Input: part model. Units: mm. Frame: model coordinates. A direction names the side the tool comes from. Round coordinates to 2 decimals unless told otherwise and drop trailing zeros. Order: outer loops, then holes, each group sorted by start corner. A loop starts at its lowest first (then second) coordinate and runs counter-clockwise, first axis right, second up. Notation, with made-up numbers: (-34, 25) -> (3, 25) arc R21 ccw to (3, 57) -> close; hole circle Ø1 at (-14, 8). An arc over 180 degrees is marked (long way). Use a Markdown table: item, result.
from build123d import *

# Parameters (mm, degrees)
SKETCH1_W           = 125
SKETCH1_H           = 60
SKETCH1_R           = 2.8
SKETCH1_R_2         = 3.25
SKETCH1_R_3         = 2.75
BOSS_EXTRUDE1_DEPTH = 30
CUT_EXTRUDE1_DEPTH  = 15
SKETCH3_R           = 3.25
CUT_EXTRUDE2_DEPTH  = 19
BOSS_EXTRUDE2_DEPTH = 5
BOSS_EXTRUDE3_REACH = 143.863
SKETCH5_W           = 6
SKETCH5_H           = 60
SKETCH5_H_2         = 17.5
SKETCH5_H_3         = 7.275
SKETCH5_W_2         = 3
SKETCH5_W_3         = 10
SKETCH5_H_4         = 15
CUT_EXTRUDE3_DEPTH  = 148.564392724
SKETCH7_W           = 23
SKETCH7_H           = 18
BOSS_EXTRUDE4_DEPTH = 12.5
SKETCH8_R           = 3.25
CUT_EXTRUDE4_DEPTH  = 129.082004981
SKETCH9_R           = 2.7
SKETCH9_W           = 24
SKETCH9_H           = 15.5
SKETCH9_W_2         = 46
BOSS_EXTRUDE5_DEPTH = 5
SKETCH10_R          = 2.7
BOSS_EXTRUDE6_DEPTH = 5
SKETCH11_R          = 2.6
CUT_EXTRUDE5_DEPTH  = 158.877325794
SKETCH12_R          = 3.5
SKETCH12_R_2        = 2.8
BOSS_EXTRUDE7_DEPTH = 0.75
FILLET1_R           = 0.75


with BuildPart() as part:
    # Sketch1 → Boss-Extrude1 (new body)
    with BuildSketch(Plane.XY):
        with Locations((-62.5, 30)):
            Rectangle(SKETCH1_W, SKETCH1_H)
        with Locations((-42.5, 42.725)):
            Circle(SKETCH1_R, mode=Mode.SUBTRACT)
        with Locations((-22, 30)):
            Circle(SKETCH1_R, mode=Mode.SUBTRACT)
        with Locations((-15, 45)):
            Circle(SKETCH1_R_2, mode=Mode.SUBTRACT)
        with Locations((-15, 15)):
            Circle(SKETCH1_R_2, mode=Mode.SUBTRACT)
        with Locations((-115, 15)):
            Circle(SKETCH1_R_3, mode=Mode.SUBTRACT)
        with Locations((-115, 45)):
            Circle(SKETCH1_R_3, mode=Mode.SUBTRACT)
    extrude(amount=BOSS_EXTRUDE1_DEPTH)

    # Sketch2 → Cut-Extrude1 (cut)
    with BuildSketch(Plane.XY.offset(30)):
        with BuildLine():
            Line((0, 0), (-22.5, 0))
            Line((-22.5, 0), (-22.5, 17.5))
            ThreePointArc((-22.5, 17.5), (-21.035533906, 21.035533906), (-17.5, 22.5))
            Line((-17.5, 22.5), (0, 22.5))
            Line((0, 22.5), (0, 0))
        make_face()
        with BuildLine():
            Line((0, 60), (-22.5, 60))
            Line((-22.5, 60), (-22.5, 42.5))
            ThreePointArc((-22.5, 42.5), (-21.035533906, 38.964466094), (-17.5, 37.5))
            Line((-17.5, 37.5), (0, 37.5))
            Line((0, 37.5), (0, 60))
        make_face()
        with BuildLine():
            Line((-107.5, 60), (-107.5, 42.5))
            ThreePointArc((-107.5, 42.5), (-108.964466094, 38.964466094), (-112.5, 37.5))
            Line((-112.5, 37.5), (-125, 37.5))
            Line((-125, 37.5), (-125, 60))
            Line((-125, 60), (-107.5, 60))
        make_face()
        with BuildLine():
            Line((-125, 0), (-107.5, 0))
            Line((-107.5, 0), (-107.5, 17.5))
            ThreePointArc((-107.5, 17.5), (-108.964466094, 21.035533906), (-112.5, 22.5))
            Line((-112.5, 22.5), (-125, 22.5))
            Line((-125, 22.5), (-125, 0))
        make_face()
    extrude(amount=-CUT_EXTRUDE1_DEPTH, mode=Mode.SUBTRACT)

    # Sketch3 → Cut-Extrude2 (cut)
    with BuildSketch(Plane(origin=(0, 0, 0), x_dir=(-1, 0, 0), z_dir=(0, 0, -1))):
        with Locations((22, 30)):
            Circle(SKETCH3_R)
        with Locations((42.5, 42.725)):
            Circle(SKETCH3_R)
    extrude(amount=-CUT_EXTRUDE2_DEPTH, mode=Mode.SUBTRACT)


with BuildPart() as body_2:
    # Sketch4 → Boss-Extrude2 (new body)
    with BuildSketch(Plane.XY.offset(45.5)):
        with BuildLine():
            Line((-107.5, 60), (-107.5, 0))
            Line((-107.5, 0), (-22.5, 0))
            Line((-22.5, 0), (-22.5, 17.5))
            ThreePointArc((-22.5, 17.5), (-21.035533906, 21.035533906), (-17.5, 22.5))
            Line((-17.5, 22.5), (0, 22.5))
            Line((0, 22.5), (0, 37.5))
            Line((0, 37.5), (-17.5, 37.5))
            ThreePointArc((-17.5, 37.5), (-21.035533906, 38.964466094), (-22.5, 42.5))
            Line((-22.5, 42.5), (-22.5, 60))
            Line((-22.5, 60), (-107.5, 60))
        make_face()
    extrude(amount=BOSS_EXTRUDE2_DEPTH)

    # Sketch5 → Boss-Extrude3 (add, up to next)
    with BuildSketch(Plane.XY.offset(30), mode=Mode.PRIVATE) as boss_extrude3_sk1:
        with Locations((-104.5, 30)):
            Rectangle(SKETCH5_W, SKETCH5_H)
    boss_extrude3_tool1 = extrude(boss_extrude3_sk1.sketch, amount=BOSS_EXTRUDE3_REACH, mode=Mode.PRIVATE) - body_2.part
    # Sketch5 → Boss-Extrude3 (add, up to next)
    with BuildSketch(Plane.XY.offset(30), mode=Mode.PRIVATE) as boss_extrude3_sk2:
        with Locations((-25.5, 8.75)):
            Rectangle(SKETCH5_W, SKETCH5_H_2)
    boss_extrude3_tool2 = extrude(boss_extrude3_sk2.sketch, amount=BOSS_EXTRUDE3_REACH, mode=Mode.PRIVATE) - body_2.part
    # Sketch5 → Boss-Extrude3 (add, up to next)
    with BuildSketch(Plane.XY.offset(30), mode=Mode.PRIVATE) as boss_extrude3_sk3:
        with Locations((-25.5, 51.25)):
            Rectangle(SKETCH5_W, SKETCH5_H_2)
    boss_extrude3_tool3 = extrude(boss_extrude3_sk3.sketch, amount=BOSS_EXTRUDE3_REACH, mode=Mode.PRIVATE) - body_2.part
    # Sketch5 → Boss-Extrude3 (add, up to next)
    with BuildSketch(Plane.XY.offset(30), mode=Mode.PRIVATE) as boss_extrude3_sk4:
        with Locations((-55.5, 56.3625)):
            Rectangle(SKETCH5_W, SKETCH5_H_3)
    boss_extrude3_tool4 = extrude(boss_extrude3_sk4.sketch, amount=BOSS_EXTRUDE3_REACH, mode=Mode.PRIVATE) - body_2.part
    # Sketch5 → Boss-Extrude3 (add, up to next)
    with BuildSketch(Plane.XY.offset(30), mode=Mode.PRIVATE) as boss_extrude3_sk5:
        with Locations((-54, 8.75)):
            Rectangle(SKETCH5_W_2, SKETCH5_H_2)
    boss_extrude3_tool5 = extrude(boss_extrude3_sk5.sketch, amount=BOSS_EXTRUDE3_REACH, mode=Mode.PRIVATE) - body_2.part
    # Sketch5 → Boss-Extrude3 (add, up to next)
    with BuildSketch(Plane.XY.offset(30), mode=Mode.PRIVATE) as boss_extrude3_sk6:
        with Locations((-5, 30)):
            Rectangle(SKETCH5_W_3, SKETCH5_H_4)
    boss_extrude3_tool6 = extrude(boss_extrude3_sk6.sketch, amount=BOSS_EXTRUDE3_REACH, mode=Mode.PRIVATE) - body_2.part

    add(part.part)  # Boss-Extrude3 merges part
    add(boss_extrude3_tool1.solids().sort_by_distance((-104.5, 30, 30))[0])
    add(boss_extrude3_tool2.solids().sort_by_distance((-25.5, 8.75, 30))[0])
    add(boss_extrude3_tool3.solids().sort_by_distance((-25.5, 51.25, 30))[0])
    add(boss_extrude3_tool4.solids().sort_by_distance((-55.5, 56.3625, 30))[0])
    add(boss_extrude3_tool5.solids().sort_by_distance((-54, 8.75, 30))[0])
    add(boss_extrude3_tool6.solids().sort_by_distance((-5, 30, 30))[0])

    # Sketch6 → Cut-Extrude3 (cut, through all)
    with BuildSketch(Plane.XY.offset(50.5)):
        with BuildLine():
            Line((-82.5, 41.5), (-75.5, 41.5))
            ThreePointArc((-75.5, 41.5), (-64, 30), (-75.5, 18.5))
            Line((-75.5, 18.5), (-82.5, 18.5))
            ThreePointArc((-82.5, 18.5), (-94, 30), (-82.5, 41.5))
        make_face()
        with BuildLine():
            Line((-91, 43.75), (-98, 43.75))
            ThreePointArc((-98, 43.75), (-99.75, 45.5), (-98, 47.25))
            Line((-98, 47.25), (-91, 47.25))
            ThreePointArc((-91, 47.25), (-89.25, 45.5), (-91, 43.75))
        make_face()
        with BuildLine():
            Line((-67, 47.25), (-60, 47.25))
            ThreePointArc((-60, 47.25), (-58.25, 45.5), (-60, 43.75))
            Line((-60, 43.75), (-67, 43.75))
            ThreePointArc((-67, 43.75), (-68.75, 45.5), (-67, 47.25))
        make_face()
        with BuildLine():
            Line((-91, 12.75), (-98, 12.75))
            ThreePointArc((-98, 12.75), (-99.75, 14.5), (-98, 16.25))
            Line((-98, 16.25), (-91, 16.25))
            ThreePointArc((-91, 16.25), (-89.25, 14.5), (-91, 12.75))
        make_face()
        with BuildLine():
            Line((-67, 16.25), (-60, 16.25))
            ThreePointArc((-60, 16.25), (-58.25, 14.5), (-60, 12.75))
            Line((-60, 12.75), (-67, 12.75))
            ThreePointArc((-67, 12.75), (-68.75, 14.5), (-67, 16.25))
        make_face()
    extrude(amount=-CUT_EXTRUDE3_DEPTH, mode=Mode.SUBTRACT)

    # Sketch7 → Boss-Extrude4 (add)
    with BuildSketch(Plane.XY.offset(50.5)):
        with Locations((-42.5, 30)):
            Rectangle(SKETCH7_W, SKETCH7_H)
    extrude(amount=BOSS_EXTRUDE4_DEPTH)

    # Sketch8 → Cut-Extrude4 (cut, through all)
    with BuildSketch(Plane(origin=(-31, 0, 0), x_dir=(0, 0, -1), z_dir=(1, 0, 0))):
        with Locations((-56.5, 30)):
            Circle(SKETCH8_R)
    extrude(amount=-CUT_EXTRUDE4_DEPTH, mode=Mode.SUBTRACT)

    # Sketch9 → Boss-Extrude5 (add)
    with BuildSketch(Plane.XZ):
        Polygon((-125, 15), (-107.5, 15), (-107.5, 50.5), (-22.5, 50.5), (-22.5, 15), (0, 15), (0, -30), (-125, -30), align=None)
        with Locations((-110, -15)):
            Circle(SKETCH9_R, mode=Mode.SUBTRACT)
        with Locations((-80, -15)):
            Circle(SKETCH9_R, mode=Mode.SUBTRACT)
        with Locations((-45, -15)):
            Circle(SKETCH9_R, mode=Mode.SUBTRACT)
        with Locations((-15, -15)):
            Circle(SKETCH9_R, mode=Mode.SUBTRACT)
        with Locations((-40.5, 37.75)):
            Rectangle(SKETCH9_W, SKETCH9_H, mode=Mode.SUBTRACT)
        with Locations((-78.5, 37.75)):
            Rectangle(SKETCH9_W_2, SKETCH9_H, mode=Mode.SUBTRACT)
    extrude(amount=BOSS_EXTRUDE5_DEPTH)

    # Sketch10 → Boss-Extrude6 (add)
    with BuildSketch(Plane(origin=(0, 0, 0), x_dir=(0, 0, -1), z_dir=(1, 0, 0))):
        Polygon((-50.5, 37.5), (-50.5, 22.5), (-15, 22.5), (-15, -5), (30, -5), (30, 60), (-15, 60), (-15, 37.5), align=None)
        with Locations((15, 45)):
            Circle(SKETCH10_R, mode=Mode.SUBTRACT)
        with Locations((15, 15)):
            Circle(SKETCH10_R, mode=Mode.SUBTRACT)
    extrude(amount=BOSS_EXTRUDE6_DEPTH)

    # Sketch11 → Cut-Extrude5 (cut, through all)
    with BuildSketch(Plane(origin=(0, 0, 45.5), x_dir=(-1, 0, 0), z_dir=(0, 0, -1))):
        with Locations((42.5, 42.725)):
            Circle(SKETCH11_R)
        with Locations((22, 30)):
            Circle(SKETCH11_R)
    extrude(amount=-CUT_EXTRUDE5_DEPTH, mode=Mode.SUBTRACT)

    # Sketch12 → Boss-Extrude7 (add)
    # profile 1 of 2: a face of its own
    with BuildSketch(Plane.XY.offset(30)):
        with Locations((-22, 30)):
            Circle(SKETCH12_R)
        with Locations(Location((-22, 30, 0), (0, 0, 180))):
            Circle(SKETCH12_R_2, mode=Mode.SUBTRACT)
    # profile 2 of 2: a face of its own
    with BuildSketch(Plane.XY.offset(30)):
        with Locations((-42.5, 42.725)):
            Circle(SKETCH12_R)
        with Locations(Location((-42.5, 42.725, 0), (0, 0, 180))):
            Circle(SKETCH12_R_2, mode=Mode.SUBTRACT)
    extrude(amount=BOSS_EXTRUDE7_DEPTH)

    # Fillet1
    fillet1_edges = [body_2.edges().sort_by_distance(p)[0] for p in [
        (-25.5, 30, 30),
        (-46, 42.725, 30),
    ]]
    fillet(fillet1_edges, radius=FILLET1_R - 0.0001)  # a hair under: the kernel refuses the full size


solid = body_2.part
1) Set-up query: faces 4 (the face through (-22.5, 6, 33)), 5 (the face through (-58.5, 56, 38)), 6 (the face through (2.465, 43.966, -17.494)), 7 (the face through (-94, 43.75, 15)). Return all of +Z, -Z, +X, -X, +Y, -Y with unobstructed straight access to the full face (end or side cutting, diameter ignored); none if empty.
Answer key:
| item | result |
|---|---|
| face 4 | +Z, +X, -Y |
| face 5 | +Y, -Y |
| face 6 | +X, -X |
| face 7 | +Z, -Z |
2) Cut plane D-D on z = -20. Return loops of the section in (x, y), and give its area (3 significant figures).
Answer key:
| item | result |
|---|---|
| outline | (-125, -5) -> (5, -5) -> (5, 60) -> (0, 60) -> (0, 0) -> (-125, 0) -> close |
| area | 950 mm^2 |
3) Draft query along Y for faces 1 (the face through (-21.815, 32.794, 24.793)), 2 (the face through (-21.07, 39, 22.6)), 3 (the face through (-116, 9, 15)). Return one class per face: released by +Y, released by -Y, zero draft, split by the parting line, or undercut.
Answer key:
| item | result |
|---|---|
| face 1 | undercut |
| face 2 | released by +Y |
| face 3 | zero draft |
4) Cut plane C-C on x = -115. Return loops of the section in (y, z).
Answer key:
| item | result |
|---|---|
| outline | (-5, -30) -> (0, -30) -> (0, 0) -> (12.25, 0) -> (12.25, 15) -> (-5, 15) -> close; (17.75, 0) -> (42.25, 0) -> (42.25, 15) -> (37.5, 15) -> (37.5, 30) -> (22.5, 30) -> (22.5, 15) -> (17.75, 15) -> close; (47.75, 0) -> (60, 0) -> (60, 15) -> (47.75, 15) -> close |
5) Cut plane A-A on x = -34. Return loops of the section in (y, z), and give its area (3 significant figures).
Answer key:
| item | result |
|---|---|
| outline | (-5, -30) -> (0, -30) -> (0, 0) -> (60, 0) -> (60, 30) -> (-5, 30) -> close; (-5, 45.5) -> (60, 45.5) -> (60, 50.5) -> (39, 50.5) -> (39, 63) -> (21, 63) -> (21, 50.5) -> (-5, 50.5) -> close; hole circle Ø6.5 at (30, 56.5) |
| area | 2,620 mm^2 |
6) Contact query for flat-ended pins moving along their axis: P1, Ø12, axis at x = -14, y = 50.5, coming from the +Z side; P2, Ø5, axis at x = -108.5, y = 3, coming from the -Z side; P3, Ø2, axis at x = -23, y = 29, coming from the -Z side; P4, Ø7, axis at x = -80, z = -15, coming from the +Y side. Output: stop coordinate, or through.
Answer key:
| item | result |
|---|---|
| P1 | stops at z = 15 |
| P2 | stops at z = 0 |
| P3 | passes through |
| P4 | stops at y = 0 |
7) Cut plane B-B on x = -80. Return loops of the section in (y, z), and give its area (3 significant figures).
Answer key:
| item | result |
|---|---|
| outline | (-5, -30) -> (0, -30) -> (0, -17.7) -> (-5, -17.7) -> close; (-5, -12.3) -> (0, -12.3) -> (0, 0) -> (18.5, 0) -> (18.5, 30) -> (-5, 30) -> close; (-5, 45.5) -> (18.5, 45.5) -> (18.5, 50.5) -> (-5, 50.5) -> close; (41.5, 0) -> (60, 0) -> (60, 30) -> (41.5, 30) -> close; (41.5, 45.5) -> (60, 45.5) -> (60, 50.5) -> (41.5, 50.5) -> close |
| area | 1,590 mm^2 |
8) Ray query, probe 1 along Y at (x, z) = (-15, 3.5); probe 2 along Y at (x, z) = (2.75, -15); probe 3 along X at (y, z) = (17, 41). Return the intervals inside material, ascending.
Answer key:
| item | result |
|---|---|
| probe 1 | y = -5 to 11.75, 18.25 to 41.75, 48.25 to 60 |
| probe 2 | y = -5 to 12.3, 17.7 to 42.3, 47.7 to 60 |
| probe 3 | x = -107.5 to -101.5, -55.5 to -52.5, -28.5 to -22.5 |
